Build history of the part. All positions in model axes, mm. Face numbers are marked on the shaded views. A direction names the side the tool comes from. Give positions to 0.01 mm unless a question says otherwise; leave off trailing zeros. Order: outer loops, then holes, each group sorted by start corner. A loop starts at its lowest first (then second) coordinate and runs counter-clockwise, first axis right, second up. Notation, with made-up numbers: M -2,65.5 L 32,65.5 A29 ccw 32,94.5 Z; hole C -24,34 d4. An arc over 180 degrees is marked long. One line per item, written item: value. Start each with the question number.
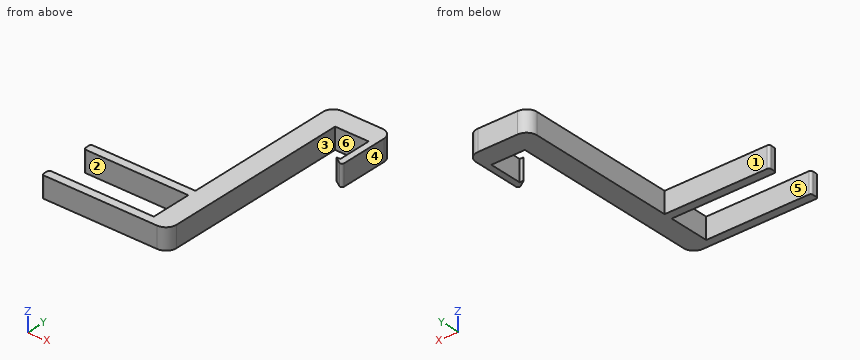
from build123d import *

# Parameters (mm, degrees)
F0_W     = 3
F0_H     = 16
F1_DEPTH = 10


with BuildPart() as f1:
    # F0 (on Top) → F1 (new body)
    with BuildSketch(Plane.XY):
        with BuildLine():
            Line((0, -23.5), (0, -19.5))
            Line((0, -19.5), (-49, -19.5))
            ThreePointArc((-49, -19.5), (-49.707107, -19.792893), (-50, -20.5))
            Line((-50, -20.5), (-50, -22.5))
            ThreePointArc((-50, -22.5), (-49.707107, -23.207107), (-49, -23.5))
            Line((-49, -23.5), (0, -23.5))
        make_face()
        with BuildLine():
            Line((0, 4), (0, 0))
            Line((0, 0), (0, -19.5))
            Line((0, -19.5), (0, -23.5))
            Line((0, -23.5), (5, -23.5))
            ThreePointArc((5, -23.5), (8.535534, -22.035534), (10, -18.5))
            Line((10, -18.5), (10, 71))
            Line((10, 71), (26, 71))
            Line((26, 71), (29, 71))
            Line((29, 71), (29, 75.97183))
            ThreePointArc((29, 75.97183), (27.535534, 79.507364), (24, 80.97183))
            Line((24, 80.97183), (5, 80.97183))
            ThreePointArc((5, 80.97183), (1.464466, 79.507364), (0, 75.97183))
            Line((0, 75.97183), (0, 4))
        make_face()
        with Locations((27.5, 63)):
            Rectangle(F0_W, F0_H)
        with BuildLine():
            Line((-48.889865, 0), (0, 0))
            Line((0, 0), (0, 4))
            Line((0, 4), (-48.962844, 4))
            ThreePointArc((-48.962844, 4), (-49.682728, 3.694094), (-49.962179, 2.963534))
            Line((-49.962179, 2.963534), (-49.889199, 0.963534))
            ThreePointArc((-49.889199, 0.963534), (-49.583959, 0.280116), (-48.889865, 0))
        make_face()
        with BuildLine():
            Line((29, 53.599753), (29, 55))
            Line((29, 55), (26, 55))
            Line((26, 55), (24.074446, 55))
            Line((24.074446, 55), (27.447859, 52.766002))
            ThreePointArc((27.447859, 52.766002), (28.473212, 52.718804), (29, 53.599753))
        make_face()
    extrude(amount=-F1_DEPTH)


solid = f1.part
1) Slice it at B-B (x = -30.5). List the corners of the cut face in (y, z).
2) Slice it at C-C (z = -2.5). List the corners of the cut face in (x, y).
3) Pull direction X, two halves, no side cores. Call the marked faces 4, 5 and 6: pulls with the +X half, pulls with the -X half, needs draft (parallel to the pull), parting line crosses it, or undercut.
4) Drill centre lines: line 1 (Y direction, x = -21.5, z = -8.5); line 2 (X direction, y = 35.5, z = -4.75); line 3 (Y direction, x = 16.5, z = -6). Where is each one in solid material? Low to high.
5) Slice it at D-D (y = -16). List the corners of the cut face in (x, z).
6) Tool access for the marked faces 1, 2 and 3: list every direction of +Z, -Z, +X, -X, +Y, -Y with a clear straight run to the whole face (end or side of a thin tool).
7) Slice it at A-A (y = 63). List the corners of the cut face in (x, z).
8) Drop flat-ended pins along their axis: P1, Ø5, axis at y = 46, z = -7.5, coming from the -X side; P2, Ø3, axis at x = -17.5, z = -3.5, coming from the +Y side; P3, Ø3, axis at x = 19.5, z = -6.5, coming from the -Y side; P4, Ø3, axis at x = 12.5, y = -4.5, coming from the +Z side. Give the stop position or say it passes through.
Results list:
1. outline: M -23.5,-10 L -19.5,-10 L -19.5,0 L -23.5,0 Z; M 0,-10 L 4,-10 L 4,0 L 0,0 Z
2. outline: M -50,-22.5 A1 ccw -49,-23.5 L 5,-23.5 A5 ccw 10,-18.5 L 10,71 L 26,71 L 26,55 L 24.07,55 L 27.45,52.77 A1 ccw 29,53.6 L 29,75.97 A5 ccw 24,80.97 L 5,80.97 A5 ccw 0,75.97 L 0,4 L -48.96,4 A1 ccw -49.96,2.96 L -49.89,0.96 A1 ccw -48.89,0 L 0,0 L 0,-19.5 L -49,-19.5 A1 ccw -50,-20.5 Z
3. face 4: pulls with the +X half
3. face 5: needs draft
3. face 6: undercut
4. line 1: y = -23.5 to -19.5, 0 to 4
4. line 2: x = 0 to 10
4. line 3: y = 71 to 80.97
5. outline: M 0,-10 L 10,-10 L 10,0 L 0,0 Z
6. face 1: +Z, -Z, -X, +Y
6. face 2: +Z, -Z, -X
6. face 3: +Z, -Z, -Y
7. outline: M 0,-10 L 10,-10 L 10,0 L 0,0 Z; M 26,-10 L 29,-10 L 29,0 L 26,0 Z
8. P1: stops at x = 0
8. P2: stops at y = 4
8. P3: stops at y = 71
8. P4: passes through
